For this review, take the finished solid that the model builds, in its own axes (mm). Give positions to 0.01 mm unless a question says otherwise; leave off trailing zeros. Order: outer loops, then holes, each group sorted by start corner. A loop starts at its lowest first (then second) coordinate and runs counter-clockwise, first axis right, second up.
Item 1: Consider section B-B (z = 5). Give the boundary of the cut face in (x, y).
Item 2: Consider section A-A (x = 14). Give the boundary of the cut face in (y, z), plus the area to 3 significant figures.
Item 3: For probe 1 along Z at (x, y) = (-15, -2); probe 2 along X at (y, z) = (-1.85, -14.5); probe 3 along X at (y, z) = (-1.35, 5.5), list the stretches that pass through material, from the lowest coordinate up.
```python
from build123d import *

# Parameters (mm, degrees)
F2_DEPTH = 2.54
F1_R     = 0.381


with BuildPart() as f2:
    # F0 (on Front) → F2 (new body)
    with BuildSketch(Plane.XZ):
        with BuildLine():
            ThreePointArc((22.86, 0), (9.785629, 6.867781), (1.27, 18.933834))
            ThreePointArc((1.27, 18.933834), (0.570733, 20.876128), (0, 22.86))
            ThreePointArc((0, 22.86), (-8.432114, 8.432114), (-22.86, 0))
            ThreePointArc((-22.86, 0), (-8.650747, -8.650747), (0, -22.86))
            ThreePointArc((0, -22.86), (8.390302, -8.390302), (22.86, 0))
        make_face()
        with BuildLine():
            ThreePointArc((1.27, -12.210841), (0.320191, -15.571962), (0, -19.05))
            ThreePointArc((0, -19.05), (-0.320191, -15.571962), (-1.27, -12.210841))
            ThreePointArc((-1.27, -12.210841), (-8.265369, -3.346681), (-19.05, 0))
            ThreePointArc((-19.05, 0), (-8.265369, 3.346681), (-1.27, 12.210841))
            ThreePointArc((-1.27, 12.210841), (-0.320191, 15.571962), (0, 19.05))
            ThreePointArc((0, 19.05), (0.320191, 15.571962), (1.27, 12.210841))
            ThreePointArc((1.27, 12.210841), (8.265369, 3.346681), (19.05, 0))
            ThreePointArc((19.05, 0), (8.265369, -3.346681), (1.27, -12.210841))
        make_face(mode=Mode.SUBTRACT)
    extrude(amount=F2_DEPTH)

    # F1
    f1_edges = [f2.edges().sort_by_distance(p)[0] for p in [
        (0, -1.27, 22.86),
        (22.86, -1.27, 0),
        (0, -1.27, -22.86),
        (-22.86, -1.27, 0),
    ]]
    fillet(f1_edges, radius=F1_R)


solid = f2.part
```
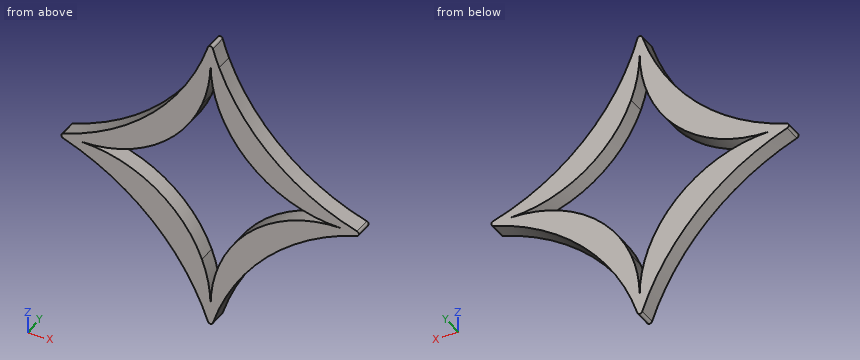
Resolved:
1. outline: (-12.47, -2.54) - (-6.19, -2.54) - (-6.19, 0) - (-12.47, 0) - close; (6.19, -2.54) - (12.13, -2.54) - (12.13, 0) - (6.19, 0) - close
2. outline: (-2.54, -3.9) - (0, -3.9) - (0, -0.68) - (-2.54, -0.68) - close; (-2.54, 0.68) - (0, 0.68) - (0, 3.75) - (-2.54, 3.75) - close
2. area: 16.0 mm2
3. probe 1: z = -3.62 to -0.44, 0.44 to 3.35
3. probe 2: x = -3.94 to -0.55, 0.55 to 3.59
3. probe 3: x = -11.79 to -5.66, 5.66 to 11.46
